```python
from build123d import *

# Parameters (mm, degrees)
SKETCH1_W                                     = 90
SKETCH1_H                                     = 50
BOSS_EXTRUDE2_DEPTH                           = 5
FILLET1_R                                     = 3
CBORE_FOR_M3_HEX_HEAD_MACHINE_SCREW1_AT_COUNT = 2
CBORE_FOR_M3_HEX_HEAD_MACHINE_SCREW1_AT_PITCH = 30
CBORE_FOR_M3_HEX_HEAD_MACHINE_SCREW1_2_COUNT  = 2
CBORE_FOR_M3_HEX_HEAD_MACHINE_SCREW1_2_PITCH  = 76.157731059
CBORE_FOR_M3_HEX_HEAD_MACHINE_SCREW1_3_COUNT  = 2
CBORE_FOR_M3_HEX_HEAD_MACHINE_SCREW1_3_PITCH  = 70


with BuildPart() as part:
    # Sketch1 → Boss-Extrude2 (new body)
    with BuildSketch(Plane(origin=(0, 0, 0), x_dir=(1, 0, 0), z_dir=(0, 1, 0))):
        Rectangle(SKETCH1_W, SKETCH1_H)
    extrude(amount=BOSS_EXTRUDE2_DEPTH)

    # Fillet1
    fillet1_edges = [part.edges().sort_by_distance(p)[0] for p in [
        (-45, 2.5, -25),
        (45, 2.5, -25),
        (45, 2.5, 25),
        (-45, 2.5, 25),
    ]]
    fillet(fillet1_edges, radius=FILLET1_R)

    # Sketch6 → CBORE for M3 Hex Head Machine Screw1 (revolve, cut)
    with BuildSketch(Plane(origin=(-35, 5, -15), x_dir=(0, 0, 1), z_dir=(1, 0, 0))):
        Polygon((0, 0), (0, 5.96137699), (1.6, 5), (1.6, 2.3), (4.2, 2.3), (4.2, 0.025), (4.225, 0), align=None)
    cbore_for_m3_hex_head_machine_screw1 = revolve(axis=Axis((-35, 11.35, -15), (0, -1, 0)), mode=Mode.SUBTRACT)

    # CBORE for M3 Hex Head Machine Screw1 at: CBORE for M3 Hex Head Machine Screw1 ×2
    with Locations(*[(0, 0, i * CBORE_FOR_M3_HEX_HEAD_MACHINE_SCREW1_AT_PITCH) for i in range(1, CBORE_FOR_M3_HEX_HEAD_MACHINE_SCREW1_AT_COUNT)]):
        add(cbore_for_m3_hex_head_machine_screw1, mode=Mode.SUBTRACT)

    # CBORE for M3 Hex Head Machine Screw1 2: CBORE for M3 Hex Head Machine Screw1 ×2
    with Locations(*[Vector(0.9191450300180579, 0, 0.3939192985791677) * (i * CBORE_FOR_M3_HEX_HEAD_MACHINE_SCREW1_2_PITCH) for i in range(1, CBORE_FOR_M3_HEX_HEAD_MACHINE_SCREW1_2_COUNT)]):
        add(cbore_for_m3_hex_head_machine_screw1, mode=Mode.SUBTRACT)

    # CBORE for M3 Hex Head Machine Screw1 3: CBORE for M3 Hex Head Machine Screw1 ×2
    with Locations(*[(i * CBORE_FOR_M3_HEX_HEAD_MACHINE_SCREW1_3_PITCH, 0, 0) for i in range(1, CBORE_FOR_M3_HEX_HEAD_MACHINE_SCREW1_3_COUNT)]):
        add(cbore_for_m3_hex_head_machine_screw1, mode=Mode.SUBTRACT)


solid = part.part
```
Input: part model. Units: mm. Frame: model coordinates. A direction names the side the tool comes from. Coordinates: 2 decimals unless noted, no trailing zeros. Order: outer loops, then holes, each group sorted by start corner. A loop starts at its lowest first (then second) coordinate and runs counter-clockwise, first axis right, second up. Notation, with made-up numbers: (-29, -1.75) - (-12, -1.75) arc R24 cw to (-12, 25.25) - close; hole circle Ø8 at (-17, 36.5). An arc over 180 degrees is marked (long way). Put each result on its own line as item: value.
1. Cut plane C-C on z = -15. Return the cut outline in (x, y) (3 decimals), then the cut area to 3 significant figures.
Report:
outline: (-45, 0) - (-36.6, 0) - (-36.6, 2.7) - (-39.2, 2.7) - (-39.2, 4.975) - (-39.225, 5) - (-45, 5) - close; (-33.4, 0) - (33.4, 0) - (33.4, 2.7) - (30.8, 2.7) - (30.8, 4.975) - (30.775, 5) - (-30.775, 5) - (-30.8, 4.975) - (-30.8, 2.7) - (-33.4, 2.7) - close; (36.6, 0) - (45, 0) - (45, 5) - (39.225, 5) - (39.2, 4.975) - (39.2, 2.7) - (36.6, 2.7) - close
area: 394 mm2
2. Draft query along Z for faces 1 (the face through (-45, 2, 0)), 2 (the face through (30.836, 3.853, -15.547)), 3 (the face through (-44.14, 2.54, 24.1)). Return one class per face: pulls with the +Z half, pulls with the -Z half, needs draft (parallel to the pull), parting line crosses it, or undercut.
Report:
face 1: needs draft
face 2: undercut
face 3: pulls with the +Z half
3. Contact query for flat-ended pins moving along their axis: pin 1 Ø6.5 at (x, z) = (35, 15) entering from -Y; pin 2 Ø4 at (x, z) = (36.5, -15) entering from +Y. Output: stop coordinate, or through.
Report:
pin 1: stops at y = 0
pin 2: stops at y = 2.7
4. Reachability of faces 4 (the face through (39.1, 3.85, 14.09)), 5 (the face through (-1, 2, -25)) from +Z, -Z, +X, -X, +Y, -Y: full face, straight path, thin tool, end or side. Return the list, or none.
Report:
face 4: +Y
face 5: -Z, +X, -X, +Y, -Y
5. Cut plane A-A on x = 35. Return the cut outline in (y, z) (3 decimals).
Report:
outline: (0, -25) - (5, -25) - (5, -19.225) - (4.975, -19.2) - (2.7, -19.2) - (2.7, -16.6) - (0, -16.6) - close; (0, -13.4) - (2.7, -13.4) - (2.7, -10.8) - (4.975, -10.8) - (5, -10.775) - (5, 10.775) - (4.975, 10.8) - (2.7, 10.8) - (2.7, 13.4) - (0, 13.4) - close; (0, 16.6) - (2.7, 16.6) - (2.7, 19.2) - (4.975, 19.2) - (5, 19.225) - (5, 25) - (0, 25) - close
6. Line query: line 1 along X through (y, z) = (1.2, -15); line 2 along X through (y, z) = (3.9, 15); line 3 along Y through (x, z) = (38.5, 15). Output: solid intervals per line, ascending.
Report:
line 1: x = -45 to -36.6, -33.4 to 33.4, 36.6 to 45
line 2: x = -45 to -39.2, -30.8 to 30.8, 39.2 to 45
line 3: y = 0 to 2.7
7. Cut plane B-B on y = 3.6. Return the cut outline in (x, z), then the cut area to 3 significant figures.
Report:
outline: (-45, -22) arc R3 ccw to (-42, -25) - (42, -25) arc R3 ccw to (45, -22) - (45, 22) arc R3 ccw to (42, 25) - (-42, 25) arc R3 ccw to (-45, 22) - close; hole circle Ø8.4 at (-35, -15); hole circle Ø8.4 at (-35, 15); hole circle Ø8.4 at (35, -15); hole circle Ø8.4 at (35, 15)
area: 4,270 mm2
